from build123d import *

# Parameters (mm, degrees)
SKETCH1_R           = 1.5
BOSS_EXTRUDE1_DEPTH = 2


with BuildPart() as part:
    # Sketch1 → Boss-Extrude1 (new body)
    with BuildSketch(Plane(origin=(0, 0, 0), x_dir=(1, 0, 0), z_dir=(0, 1, 0))):
        with BuildLine():
            ThreePointArc((-102.071067812, 110.942475232), (-108.071067812, 108.071067812), (-110.942475232, 102.071067812))
            ThreePointArc((-110.942475232, 102.071067812), (-110.02026395, 98.825326817), (-108.071067812, 96.071067812))
            Line((-108.071067812, 96.071067812), (-94.262265521, 82.262265521))
            ThreePointArc((-94.262265521, 82.262265521), (-92.094538008, 79.018032033), (-91.333333333, 75.19119771))
            Line((-91.333333333, 75.19119771), (-91.333333333, 73.475468957))
            ThreePointArc((-91.333333333, 73.475468957), (-92.094538008, 69.648634633), (-94.262265521, 66.404401145))
            Line((-94.262265521, 66.404401145), (-108.071067812, 52.595598855))
            ThreePointArc((-108.071067812, 52.595598855), (-110.238795325, 49.351365367), (-111, 45.524531043))
            Line((-111, 45.524531043), (-111, 33.80880229))
            ThreePointArc((-111, 33.80880229), (-110.238795325, 29.981967967), (-108.071067812, 26.737734479))
            Line((-108.071067812, 26.737734479), (-94.262265521, 12.928932188))
            ThreePointArc((-94.262265521, 12.928932188), (-92.094538008, 9.6846987), (-91.333333333, 5.857864376))
            Line((-91.333333333, 5.857864376), (-91.333333333, -5.857864376))
            ThreePointArc((-91.333333333, -5.857864376), (-92.094538008, -9.6846987), (-94.262265521, -12.928932188))
            Line((-94.262265521, -12.928932188), (-108.071067812, -26.737734479))
            ThreePointArc((-108.071067812, -26.737734479), (-110.238795325, -29.981967967), (-111, -33.80880229))
            Line((-111, -33.80880229), (-111, -45.524531043))
            ThreePointArc((-111, -45.524531043), (-110.238795325, -49.351365367), (-108.071067812, -52.595598855))
            Line((-108.071067812, -52.595598855), (-94.262265521, -66.404401145))
            ThreePointArc((-94.262265521, -66.404401145), (-92.094538008, -69.648634633), (-91.333333333, -73.475468957))
            Line((-91.333333333, -73.475468957), (-91.333333333, -75.19119771))
            ThreePointArc((-91.333333333, -75.19119771), (-92.094538008, -79.018032033), (-94.262265521, -82.262265521))
            Line((-94.262265521, -82.262265521), (-108.071067812, -96.071067812))
            ThreePointArc((-108.071067812, -96.071067812), (-110.02026395, -98.825326817), (-110.942475232, -102.071067812))
            ThreePointArc((-110.942475232, -102.071067812), (-108.071067812, -108.071067812), (-102.071067812, -110.942475232))
            ThreePointArc((-102.071067812, -110.942475232), (-98.825326817, -110.02026395), (-96.071067812, -108.071067812))
            Line((-96.071067812, -108.071067812), (-75.428932188, -87.428932188))
            ThreePointArc((-75.428932188, -87.428932188), (-72.1846987, -85.261204675), (-68.357864376, -84.5))
            Line((-68.357864376, -84.5), (68.357864376, -84.5))
            ThreePointArc((68.357864376, -84.5), (72.1846987, -85.261204675), (75.428932188, -87.428932188))
            Line((75.428932188, -87.428932188), (96.071067812, -108.071067812))
            ThreePointArc((96.071067812, -108.071067812), (98.825326817, -110.02026395), (102.071067812, -110.942475232))
            ThreePointArc((102.071067812, -110.942475232), (108.071067812, -108.071067812), (110.942475232, -102.071067812))
            ThreePointArc((110.942475232, -102.071067812), (110.02026395, -98.825326817), (108.071067812, -96.071067812))
            Line((108.071067812, -96.071067812), (94.262265521, -82.262265521))
            ThreePointArc((94.262265521, -82.262265521), (92.094538008, -79.018032033), (91.333333333, -75.19119771))
            Line((91.333333333, -75.19119771), (91.333333333, -73.475468957))
            ThreePointArc((91.333333333, -73.475468957), (92.094538008, -69.648634633), (94.262265521, -66.404401145))
            Line((94.262265521, -66.404401145), (108.071067812, -52.595598855))
            ThreePointArc((108.071067812, -52.595598855), (110.238795325, -49.351365367), (111, -45.524531043))
            Line((111, -45.524531043), (111, -33.80880229))
            ThreePointArc((111, -33.80880229), (110.238795325, -29.981967967), (108.071067812, -26.737734479))
            Line((108.071067812, -26.737734479), (94.262265521, -12.928932188))
            ThreePointArc((94.262265521, -12.928932188), (92.094538008, -9.6846987), (91.333333333, -5.857864376))
            Line((91.333333333, -5.857864376), (91.333333333, 5.857864376))
            ThreePointArc((91.333333333, 5.857864376), (92.094538008, 9.6846987), (94.262265521, 12.928932188))
            Line((94.262265521, 12.928932188), (108.071067812, 26.737734479))
            ThreePointArc((108.071067812, 26.737734479), (110.238795325, 29.981967967), (111, 33.80880229))
            Line((111, 33.80880229), (111, 45.524531043))
            ThreePointArc((111, 45.524531043), (110.238795325, 49.351365367), (108.071067812, 52.595598855))
            Line((108.071067812, 52.595598855), (94.262265521, 66.404401145))
            ThreePointArc((94.262265521, 66.404401145), (92.094538008, 69.648634633), (91.333333333, 73.475468957))
            Line((91.333333333, 73.475468957), (91.333333333, 75.19119771))
            ThreePointArc((91.333333333, 75.19119771), (92.094538008, 79.018032033), (94.262265521, 82.262265521))
            Line((94.262265521, 82.262265521), (108.071067812, 96.071067812))
            ThreePointArc((108.071067812, 96.071067812), (110.02026395, 98.825326817), (110.942475232, 102.071067812))
            ThreePointArc((110.942475232, 102.071067812), (108.071067812, 108.071067812), (102.071067812, 110.942475232))
            ThreePointArc((102.071067812, 110.942475232), (98.825326817, 110.02026395), (96.071067812, 108.071067812))
            Line((96.071067812, 108.071067812), (75.428932188, 87.428932188))
            ThreePointArc((75.428932188, 87.428932188), (72.1846987, 85.261204675), (68.357864376, 84.5))
            Line((68.357864376, 84.5), (-68.357864376, 84.5))
            ThreePointArc((-68.357864376, 84.5), (-72.1846987, 85.261204675), (-75.428932188, 87.428932188))
            Line((-75.428932188, 87.428932188), (-96.071067812, 108.071067812))
            ThreePointArc((-96.071067812, 108.071067812), (-98.825326817, 110.02026395), (-102.071067812, 110.942475232))
        make_face()
        with Locations(Location((-104.5, -104.5, 0), (0, 0, 270))):
            Circle(SKETCH1_R, mode=Mode.SUBTRACT)
        with Locations(Location((-84.5, -39.666666667, 0), (0, 0, 270))):
            Circle(SKETCH1_R, mode=Mode.SUBTRACT)
        with Locations(Location((-57, -39.666666667, 0), (0, 0, 270))):
            Circle(SKETCH1_R, mode=Mode.SUBTRACT)
        with BuildLine():
            ThreePointArc((-63.797799427, 13.535533906), (-62.175682683, 14.619397663), (-60.262265521, 15))
            Line((-60.262265521, 15), (-56.404401145, 15))
            ThreePointArc((-56.404401145, 15), (-54.490983983, 14.619397663), (-52.868867239, 13.535533906))
            Line((-52.868867239, 13.535533906), (-44.797799427, 5.464466094))
            ThreePointArc((-44.797799427, 5.464466094), (-43.713935671, 3.84234935), (-43.333333333, 1.928932188))
            Line((-43.333333333, 1.928932188), (-43.333333333, -1.928932188))
            ThreePointArc((-43.333333333, -1.928932188), (-43.713935671, -3.84234935), (-44.797799427, -5.464466094))
            Line((-44.797799427, -5.464466094), (-52.868867239, -13.535533906))
            ThreePointArc((-52.868867239, -13.535533906), (-54.490983983, -14.619397663), (-56.404401145, -15))
            Line((-56.404401145, -15), (-60.262265521, -15))
            ThreePointArc((-60.262265521, -15), (-62.175682683, -14.619397663), (-63.797799427, -13.535533906))
            Line((-63.797799427, -13.535533906), (-71.868867239, -5.464466094))
            ThreePointArc((-71.868867239, -5.464466094), (-72.952730996, -3.84234935), (-73.333333333, -1.928932188))
            Line((-73.333333333, -1.928932188), (-73.333333333, 1.928932188))
            ThreePointArc((-73.333333333, 1.928932188), (-72.952730996, 3.84234935), (-71.868867239, 5.464466094))
            Line((-71.868867239, 5.464466094), (-63.797799427, 13.535533906))
        make_face(mode=Mode.SUBTRACT)
        with BuildLine():
            Line((-12.928932188, -36.5), (12.928932188, -36.5))
            ThreePointArc((12.928932188, -36.5), (14.84234935, -36.880602337), (16.464466094, -37.964466094))
            Line((16.464466094, -37.964466094), (36.464466094, -57.964466094))
            ThreePointArc((36.464466094, -57.964466094), (37.548329851, -63.413417162), (32.928932188, -66.5))
            Line((32.928932188, -66.5), (-32.928932188, -66.5))
            ThreePointArc((-32.928932188, -66.5), (-37.548329851, -63.413417162), (-36.464466094, -57.964466094))
            Line((-36.464466094, -57.964466094), (-16.464466094, -37.964466094))
            ThreePointArc((-16.464466094, -37.964466094), (-14.84234935, -36.880602337), (-12.928932188, -36.5))
        make_face(mode=Mode.SUBTRACT)
        with Locations(Location((-11, 0, 0), (0, 0, 270))):
            Circle(SKETCH1_R, mode=Mode.SUBTRACT)
        with Locations(Location((104.5, -104.5, 0), (0, 0, 270))):
            Circle(SKETCH1_R, mode=Mode.SUBTRACT)
        with Locations(Location((11, 0, 0), (0, 0, 270))):
            Circle(SKETCH1_R, mode=Mode.SUBTRACT)
        with Locations(Location((57, -39.666666667, 0), (0, 0, 270))):
            Circle(SKETCH1_R, mode=Mode.SUBTRACT)
        with Locations(Location((84.5, -39.666666667, 0), (0, 0, 270))):
            Circle(SKETCH1_R, mode=Mode.SUBTRACT)
        with BuildLine():
            Line((73.333333333, 1.928932188), (73.333333333, -1.928932188))
            ThreePointArc((73.333333333, -1.928932188), (72.952730996, -3.84234935), (71.868867239, -5.464466094))
            Line((71.868867239, -5.464466094), (63.797799427, -13.535533906))
            ThreePointArc((63.797799427, -13.535533906), (62.175682683, -14.619397663), (60.262265521, -15))
            Line((60.262265521, -15), (56.404401145, -15))
            ThreePointArc((56.404401145, -15), (54.490983983, -14.619397663), (52.868867239, -13.535533906))
            Line((52.868867239, -13.535533906), (44.797799427, -5.464466094))
            ThreePointArc((44.797799427, -5.464466094), (43.713935671, -3.84234935), (43.333333333, -1.928932188))
            Line((43.333333333, -1.928932188), (43.333333333, 1.928932188))
            ThreePointArc((43.333333333, 1.928932188), (43.713935671, 3.84234935), (44.797799427, 5.464466094))
            Line((44.797799427, 5.464466094), (52.868867239, 13.535533906))
            ThreePointArc((52.868867239, 13.535533906), (54.490983983, 14.619397663), (56.404401145, 15))
            Line((56.404401145, 15), (60.262265521, 15))
            ThreePointArc((60.262265521, 15), (62.175682683, 14.619397663), (63.797799427, 13.535533906))
            Line((63.797799427, 13.535533906), (71.868867239, 5.464466094))
            ThreePointArc((71.868867239, 5.464466094), (72.952730996, 3.84234935), (73.333333333, 1.928932188))
        make_face(mode=Mode.SUBTRACT)
        with Locations(Location((-84.5, 39.666666667, 0), (0, 0, 270))):
            Circle(SKETCH1_R, mode=Mode.SUBTRACT)
        with Locations(Location((-57, 39.666666667, 0), (0, 0, 270))):
            Circle(SKETCH1_R, mode=Mode.SUBTRACT)
        with Locations(Location((-104.5, 104.5, 0), (0, 0, 270))):
            Circle(SKETCH1_R, mode=Mode.SUBTRACT)
        with BuildLine():
            ThreePointArc((-36.464466094, 57.964466094), (-37.548329851, 63.413417162), (-32.928932188, 66.5))
            Line((-32.928932188, 66.5), (32.928932188, 66.5))
            ThreePointArc((32.928932188, 66.5), (37.548329851, 63.413417162), (36.464466094, 57.964466094))
            Line((36.464466094, 57.964466094), (16.464466094, 37.964466094))
            ThreePointArc((16.464466094, 37.964466094), (14.84234935, 36.880602337), (12.928932188, 36.5))
            Line((12.928932188, 36.5), (-12.928932188, 36.5))
            ThreePointArc((-12.928932188, 36.5), (-14.84234935, 36.880602337), (-16.464466094, 37.964466094))
            Line((-16.464466094, 37.964466094), (-36.464466094, 57.964466094))
        make_face(mode=Mode.SUBTRACT)
        with Locations(Location((57, 39.666666667, 0), (0, 0, 270))):
            Circle(SKETCH1_R, mode=Mode.SUBTRACT)
        with Locations(Location((84.5, 39.666666667, 0), (0, 0, 270))):
            Circle(SKETCH1_R, mode=Mode.SUBTRACT)
        with Locations(Location((15.75, 81.5, 0), (0, 0, 270))):
            Circle(SKETCH1_R, mode=Mode.SUBTRACT)
        with Locations(Location((34.75, 81.5, 0), (0, 0, 270))):
            Circle(SKETCH1_R, mode=Mode.SUBTRACT)
        with Locations(Location((104.5, 104.5, 0), (0, 0, 270))):
            Circle(SKETCH1_R, mode=Mode.SUBTRACT)
    extrude(amount=BOSS_EXTRUDE1_DEPTH)


solid = part.part
Design review of the part built by this model. Coordinates are the model's own, in mm. A direction names the side the tool comes from. Coordinates: 2 decimals unless noted, no trailing zeros. Order: outer loops, then holes, each group sorted by start corner. A loop starts at its lowest first (then second) coordinate and runs counter-clockwise, first axis right, second up.
Item 1: The part is to be moulded in two halves that separate along Z. For faces 5 (the flat face through (-2, 0, -2)), 6 (the flat face through (67.89, 0.986, 9.444)), 7 (the cylindrical face through (-108.14, 0.99, 108)), say which applies: pulls with the +Z half, pulls with the -Z half, needs draft (parallel to the pull), parting line crosses it, or undercut.
Item 2: Take a section at D-D, the plane z = -18.5. Write out the cut boundary in (x, y), then the cut area to 3 significant figures.
Item 3: For line 1 (Z direction, x = 2.5, y = 1.9); line 2 (Z direction, x = -84.5, y = 1.2); line 3 (Z direction, x = 93.5, y = 1.4), list the stretches that pass through material, from the lowest coordinate up.
Item 4: For faces 1 (the flat face through (-101.263, 0.986, -19.93)), 2 (the flat face through (-67.777, 0.986, 9.556)), 3 (the flat face through (101.263, 0.986, -59.403)), 4 (the cylindrical face through (108.14, 0.99, -108)), list the 3-axis set-ups (+Z, -Z, +X, -X, +Y, -Y) from which the entire face can be reached by the end or side of a thin tool; tool diameter is ignored.
Item 5: For pin 1 Ø1 at (x, y) = (32.5, 1) entering from +Z; pin 2 Ø10 at (x, z) = (-59.5, -7.5) entering from +Y; pin 3 Ø0.9 at (y, z) = (1.5, 74.5) entering from +X; pin 4 Ø0.5 at (y, z) = (1, 74.5) entering from -X, all flat-tipped, find the tip position at first contact; note any pin that passes through.
Item 6: Take a section at C-C, the plane z = 21. Write out the cut boundary in (x, y), then the cut area to 3 significant figures.
Item 7: Take a section at B-B, the plane y = 1.2. Count the separate pieces of the cut face and the enclosed holes in it, then the cut area to 3 significant figures.
Item 8: Take a section at A-A, the plane x = -6.5. Write out the cut boundary in (y, z).
The answers:
1. face 5: needs draft
1. face 6: undercut
1. face 7: pulls with the +Z half
2. outline: (-99.83, 0) - (99.83, 0) - (99.83, 2) - (-99.83, 2) - close
2. area: 399 mm2
3. line 1: z = -84.5 to -66.5, -36.5 to 36.5, 66.5 to 84.5
3. line 2: z = -96.5 to -41.17, -38.17 to 38.17, 41.17 to 96.5
3. line 3: z = -105.5 to -81.41, -67.26 to -12.07, 12.07 to 67.26, 81.41 to 105.5
4. face 1: -X, +Y, -Y
4. face 2: +Y, -Y
4. face 3: +X, +Y, -Y
4. face 4: -Z, +X, +Y, -Y
5. pin 1: stops at z = 84.5
5. pin 2: passes through
5. pin 3: stops at x = 91.33
5. pin 4: stops at x = -91.33
6. outline: (-102.33, 0) - (102.33, 0) - (102.33, 2) - (-102.33, 2) - close
6. area: 409 mm2
7. separate pieces: 1
7. enclosed holes: 20
7. area: 31,300 mm2
8. outline: (0, -84.5) - (2, -84.5) - (2, -66.5) - (0, -66.5) - close; (0, -36.5) - (2, -36.5) - (2, 36.5) - (0, 36.5) - close; (0, 66.5) - (2, 66.5) - (2, 84.5) - (0, 84.5) - close
